from build123d import *

# Parameters (mm, degrees)
F0_R     = 3
F0_W     = 29.4
F0_H     = 1.2
F0_R_2   = 1.6
F1_DEPTH = 1.8
F2_DEPTH = 2


# Not quite as in the source:
# - a feature names something its author has since deleted; it is built from what else it names


with BuildPart() as f1:
    # F0 (on Front) → F1 (new body)
    with BuildSketch(Plane.XZ):
        Polygon((-14.7, 13), (-17.7, 13), (-17.7, -13), (-14.7, -13), (-14.7, -11.8), (14.7, -11.8), (14.7, -13), (17.7, -13), (17.7, 13), (14.7, 13), (14.7, 11.8), (-14.7, 11.8), align=None)
        with Locations((-6.5, 0)):
            Circle(F0_R, mode=Mode.SUBTRACT)
        with Locations((12.5, 0)):
            Circle(F0_R, mode=Mode.SUBTRACT)
        with Locations((0, 12.4)):
            Rectangle(F0_W, F0_H)
        with Locations((0, -12.4)):
            Rectangle(F0_W, F0_H)
        with Locations((-6.5, 0)):
            Circle(F0_R)
        with Locations((-6.5, 0)):
            Circle(F0_R_2, mode=Mode.SUBTRACT)
        with Locations((12.5, 0)):
            Circle(F0_R)
        with Locations((12.5, 0)):
            Circle(F0_R_2, mode=Mode.SUBTRACT)
    extrude(amount=F1_DEPTH)

    # F0 (on Front) → F2 (join)
    with BuildSketch(Plane.XZ):
        with Locations((12.5, 0)):
            Circle(F0_R)
        with Locations((12.5, 0)):
            Circle(F0_R_2, mode=Mode.SUBTRACT)
        with Locations((-6.5, 0)):
            Circle(F0_R)
        with Locations((-6.5, 0)):
            Circle(F0_R_2, mode=Mode.SUBTRACT)
        with Locations((0, 12.4)):
            Rectangle(F0_W, F0_H)
        with Locations((0, -12.4)):
            Rectangle(F0_W, F0_H)
    extrude(amount=-F2_DEPTH)


solid = f1.part
Input: part model. Units: mm. Frame: model coordinates. A direction names the side the tool comes from. Coordinates: 2 decimals unless noted, no trailing zeros. Loops run counter-clockwise (first coordinate to the right, second up) from the corner with the lowest first, then second, coordinate; pieces in that order, holes last.
(1) Section B-B on y = 1. Return the cut outline in (x, z).
(2) Section A-A on x = 12.5. Return the cut outline in (y, z), then the cut area to 3 significant figures.
(3) Pull-direction query (X, two-part tool) for faces 4 (the face through (-3.64, 0.99, 0.9)), 5 (the face through (0, 0, 13)), 6 (the face through (17.7, -1, 0)); classes: released by +X, released by -X, zero draft, split by the parting line, or undercut.
(4) First-contact query: pin 1 Ø1 at (y, z) = (1.5, 12.5) entering from -X; pin 2 Ø1.3 at (y, z) = (1, 12.5) entering from +X; pin 3 Ø2 at (x, z) = (6.5, 0.5) entering from +Y. Flat tips, straight axial feed; report the tip coordinate or a pass-through.
(5) Material intervals for probe 1 along Z at (x, y) = (12.5, 1.1); probe 2 along Z at (x, y) = (12.5, -0.9); probe 3 along Z at (x, y) = (8.5, 1.05), sorted ascending.
(6) Set-up query: faces 1 (the face through (0, 1, -11.8)), 2 (the face through (14.7, 1, -12)), 3 (the face through (-14.7, 1, -12)). Return all of +Z, -Z, +X, -X, +Y, -Y with unobstructed straight access to the full face (end or side cutting, diameter ignored); none if empty.
(7) Section C-C on z = 0. Return the cut outline in (x, y), then the cut area to 3 significant figures.
(8) Section D-D on x = 5. Return the cut outline in (y, z).
Data:
1. outline: (-14.7, -13) - (14.7, -13) - (14.7, -11.8) - (-14.7, -11.8) - close; (-14.7, 11.8) - (14.7, 11.8) - (14.7, 13) - (-14.7, 13) - close; circle Ø6 at (-6.5, 0); circle Ø6 at (12.5, 0); hole circle Ø3.2 at (-6.5, 0); hole circle Ø3.2 at (12.5, 0)
2. outline: (-1.8, -13) - (2, -13) - (2, -11.8) - (0, -11.8) - (0, -3) - (2, -3) - (2, -1.6) - (-1.8, -1.6) - close; (-1.8, 1.6) - (2, 1.6) - (2, 3) - (0, 3) - (0, 11.8) - (2, 11.8) - (2, 13) - (-1.8, 13) - close
2. area: 51.4 mm2
3. face 4: undercut
3. face 5: zero draft
3. face 6: released by +X
4. pin 1: stops at x = -14.7
4. pin 2: stops at x = 14.7
4. pin 3: stops at y = 0
5. probe 1: z = -13 to -11.8, -3 to -1.6, 1.6 to 3, 11.8 to 13
5. probe 2: z = -13 to -1.6, 1.6 to 13
5. probe 3: z = -13 to -11.8, 11.8 to 13
6. face 1: +X, -X, +Y
6. face 2: -Z, +X, +Y
6. face 3: +Z, -Z, -X, +Y
7. outline: (-17.7, -1.8) - (-8.1, -1.8) - (-8.1, 2) - (-9.5, 2) - (-9.5, 0) - (-17.7, 0) - close; (-4.9, -1.8) - (10.9, -1.8) - (10.9, 2) - (9.5, 2) - (9.5, 0) - (-3.5, 0) - (-3.5, 2) - (-4.9, 2) - close; (14.1, -1.8) - (17.7, -1.8) - (17.7, 0) - (15.5, 0) - (15.5, 2) - (14.1, 2) - close
7. area: 63.4 mm2
8. outline: (-1.8, -13) - (2, -13) - (2, -11.8) - (0, -11.8) - (0, 11.8) - (2, 11.8) - (2, 13) - (-1.8, 13) - close
